Geometry check sheet. Reference: the model listing, model coordinates, mm. A direction names the side the tool comes from. Give positions to 0.01 mm unless a question says otherwise; leave off trailing zeros. Write each loop counter-clockwise with the first axis right and the second up, starting at its lowest first coordinate (ties: lowest second). Pieces come first, ordered by that corner, then holes. Notation, with made-up numbers: (72.5, 89) -> (125.5, 89) arc R28 cw to (125.5, 117) -> close; hole circle Ø11 at (8.25, 71). An arc over 180 degrees is marked (long way). One line per item, written item: value.
Autodesk Fusion 360 part; units mm, degrees
sketch "スケッチ1" plane through (0, 0, 0) normal (0, 0, 1) x (1, 0, 0)
  line L0 (942.8497, -699.0501) -> (942.8497, -547.0501)
  line L1 (934.8497, -699.0501) -> (934.8497, -547.0501)
  line L2 (742.8497, -547.0501) -> (742.8497, -699.0501)
  line L3 (750.8497, -547.0501) -> (750.8497, -699.0501)
  line L4 (766.8497, -723.0501) -> (918.8497, -723.0501)
  line L5 (766.8497, -715.0501) -> (918.8497, -715.0501)
  arc A0 (742.8497, -699.0501) -> (766.8497, -723.0501) centre (766.8497, -699.0501) ccw
  arc A1 (750.8497, -699.0501) -> (766.8497, -715.0501) centre (766.8497, -699.0501) ccw
  arc A2 (918.8497, -723.0501) -> (942.8497, -699.0501) centre (918.8497, -699.0501) ccw
  arc A3 (918.8497, -715.0501) -> (934.8497, -699.0501) centre (918.8497, -699.0501) ccw
  line L6 (918.8497, -523.0501) -> (766.8497, -523.0501)
  line L7 (918.8497, -531.0501) -> (766.8497, -531.0501)
  arc A4 (766.8497, -523.0501) -> (742.8497, -547.0501) centre (766.8497, -547.0501) ccw
  arc A5 (766.8497, -531.0501) -> (750.8497, -547.0501) centre (766.8497, -547.0501) ccw
  arc A6 (942.8497, -547.0501) -> (918.8497, -523.0501) centre (918.8497, -547.0501) ccw
  arc A7 (934.8497, -547.0501) -> (918.8497, -531.0501) centre (918.8497, -547.0501) ccw
  point P0 (842.8497, -623.0501)
extrude "押し出し1" add sketch "スケッチ1" along normal blind 100
1) Tool access check on faces 1 (the flat face through (844, -531.05, 49)), 2 (the flat face through (842, -719, 0)). Record the directions out of +Z, -Z, +X, -X, +Y, -Y that give a thin tool (end or side, any length) a straight path to the whole face; none if there is none.
Verdict:
face 1: +Z, -Z
face 2: -Z, +X, -X, +Y, -Y
2) Sectioned sample at B-B on x = 906. Record the cut outline in (y, z), plus the area to 3 significant figures.
Verdict:
outline: (-723.05, 0) -> (-715.05, 0) -> (-715.05, 100) -> (-723.05, 100) -> close; (-531.05, 0) -> (-523.05, 0) -> (-523.05, 100) -> (-531.05, 100) -> close
area: 1,600 mm^2
3) Scan lines: probe 1 along Y at (x, z) = (778, 23.5); probe 2 along X at (y, z) = (-687, 59.5); probe 3 along Y at (x, z) = (933.5, 50.5). Record each from-to range of solid material in increasing order.
Verdict:
probe 1: -723.05 to -715.05, -531.05 to -523.05
probe 2: 742.85 to 750.85, 934.85 to 942.85
probe 3: -718.06 to -705.48, -540.62 to -528.04
4) Sectioned sample at A-A on y = -627. Record the cut outline in (x, z).
Verdict:
outline: (742.85, 0) -> (750.85, 0) -> (750.85, 100) -> (742.85, 100) -> close; (934.85, 0) -> (942.85, 0) -> (942.85, 100) -> (934.85, 100) -> close
5) Mould release check, pull along X, two halves, no side actions. Record for faces 3 (the flat face through (842, -719, 100)), 4 (the cylindrical face through (749.69, -530.27, 49.3)), 5 (the flat face through (942.85, -624, 49)), 6 (the flat face through (842, -715.05, 49)): released by +X, released by -X, zero draft, split by the parting line, or undercut.
Verdict:
face 3: zero draft
face 4: released by -X
face 5: released by +X
face 6: undercut
6) Sectioned sample at C-C on z = 40. Record the cut outline in (x, y).
Verdict:
outline: (742.85, -699.05) arc R24 ccw to (766.85, -723.05) -> (918.85, -723.05) arc R24 ccw to (942.85, -699.05) -> (942.85, -547.05) arc R24 ccw to (918.85, -523.05) -> (766.85, -523.05) arc R24 ccw to (742.85, -547.05) -> close; hole (750.85, -699.05) arc R16 ccw to (766.85, -715.05) -> (918.85, -715.05) arc R16 ccw to (934.85, -699.05) -> (934.85, -547.05) arc R16 ccw to (918.85, -531.05) -> (766.85, -531.05) arc R16 ccw to (750.85, -547.05) -> close
